from build123d import *

# Parameters (mm, degrees)
SKETCH1_R           = 7.5
SKETCH1_R_2         = 3.05
BOSS_EXTRUDE1_DEPTH = 3
CIRPATTERN1_COUNT   = 10


with BuildPart() as part:
    # Sketch1 → Boss-Extrude1 (new body)
    with BuildSketch(Plane(origin=(0, 0, 0), x_dir=(1, 0, 0), z_dir=(0, 1, 0))):
        with Locations(Location((0, 0, 0), (0, 0, 270))):
            Circle(SKETCH1_R)
        with Locations(Location((0, 0, 0), (0, 0, 270))):
            Circle(SKETCH1_R_2, mode=Mode.SUBTRACT)
    extrude(amount=BOSS_EXTRUDE1_DEPTH)

    # Sketch3 → Revolve2 (revolve)
    with BuildSketch(Plane(origin=(0, 0, 0), x_dir=(0, 0, -1), z_dir=(1, 0, 0))):
        with BuildLine():
            Line((4.35, 0), (5.75, 0))
            ThreePointArc((5.75, 0), (5.05, -0.7), (4.35, 0))
        make_face()
    revolve2 = revolve(axis=Axis((0, 0, -8.25), (0, 0, 1)))

    # CirPattern1: Revolve2 ×10 about axis
    cirpattern1_axis = Axis((0, 0, 0), (0, 1, 0))
    for i in range(1, CIRPATTERN1_COUNT):
        add(revolve2.rotate(cirpattern1_axis, i * 360 / CIRPATTERN1_COUNT))


solid = part.part
Can you work these out from the model? Positions are in its coordinate system, mm. Give positions to 0.01 mm unless a question says otherwise; leave off trailing zeros. Write each loop counter-clockwise with the first axis right and the second up, starting at its lowest first coordinate (ties: lowest second). Pieces come first, ordered by that corner, then holes. Notation, with made-up numbers: (20, 82) -> (64, 82) arc R22 cw to (64, 109) -> close; hole circle Ø2 at (88.25, 24.5). An arc over 180 degrees is marked (long way). Answer as a JSON object with one key per item and string values. Group by question number.
Item 1: Suppose I cut it at C-C (y = 2.05). Please give me the cut outline in (x, z).
Item 2: Suppose I cut it at B-B (z = 0). Please give me the cut outline in (x, y), plus the area to 3 significant figures.
Item 3: We'd pull the mould along X, two halves only. Please class faces 1 (the face through (0.33, 1.479, -7.493)), 2 (the face through (0.1, 3, 3.2)), 3 (the face through (0.1, 0, 3.2)): +X half, -X half, draft (parallel to the pull), parting line (faces both ways), or undercut.
Item 4: Suppose I cut it at A-A (x = 0). Please give me the cut outline in (y, z).
Item 5: I'm going to push flat-ended pins straight in: P1, Ø1.5, axis at y = -0.5, z = 3.5, coming from the -X side; P2, Ø8, axis at x = 0, z = 0, coming from the -Y side; P3, Ø6, axis at x = 3.5, z = -3, coming from the -Y side. Where does each tip first touch, or does it pass through?
Item 6: Please list where these lines run through material, in increasing order: line 1 (X direction, y = 1, z = 0); line 2 (Y direction, x = -4.25, z = 5); line 3 (X direction, y = -0.05, z = -1.75). Write a range as [from, to].
Item 7: Suppose I cut it at D-D (x = -2.75). Please give me the cut outline in (y, z).
Findings:
{
 "1": {"outline": "circle Ø15 at (0, 0); hole circle Ø6.1 at (0, 0)"},
 "2": {"outline": "(-7.5, 0) -> (-3.05, 0) -> (-3.05, 3) -> (-7.5, 3) -> close; (3.05, 0) -> (7.5, 0) -> (7.5, 3) -> (3.05, 3) -> close", "area": "26.7 mm²"},
 "3": {"face 1": "parting line", "face 2": "draft", "face 3": "undercut"},
 "4": {"outline": "(0, -7.5) -> (3, -7.5) -> (3, -3.05) -> (0, -3.05) -> (0, -4.35) arc R0.7 ccw to (0, -5.75) -> close; (0, 3.05) -> (3, 3.05) -> (3, 7.5) -> (0, 7.5) -> (0, 5.75) arc R0.7 ccw to (0, 4.35) -> close"},
 "5": {"P1": "stops at x = -6.9", "P2": "stops at y = 0", "P3": "stops at y = -0.7"},
 "6": {"line 1": "x = [-7.5, -3.05], [3.05, 7.5]", "line 2": "y = [0, 3]", "line 3": "x = [-5.47, -4.13], [4.13, 5.47]"},
 "7": {"outline": "(0, -6.98) -> (3, -6.98) -> (3, -1.32) -> (0, -1.32) -> (0, -3.42) arc R0.67 ccw to (0, -4.75) -> close; (0, 1.32) -> (3, 1.32) -> (3, 6.98) -> (0, 6.98) -> (0, 4.75) arc R0.67 ccw to (0, 3.42) -> close"}
}
